Read the model definition and answer for the solid it produces. Units are mm, in the model's axes. A direction names the side the tool comes from. Give positions to 0.01 mm unless a question says otherwise; leave off trailing zeros. Loops run counter-clockwise (first coordinate to the right, second up) from the corner with the lowest first, then second, coordinate; pieces in that order, holes last. Notation, with made-up numbers: (9.5, 84) - (20.5, 84) arc R4 ccw to (20.5, 89) - close; hole circle Ø8 at (1.25, -39). An arc over 180 degrees is marked (long way). Use a Markdown table: item, result. Add a question column.
Item 1: A cutting plane is placed at D-D (y = -9.75). Determine the outline of the cut face in (x, z) (3 decimals).
Item 2: Each of these flat-tipped pins is pushed along its axis until it touches: P1, Ø1.5, axis at y = -3.5, z = -13, coming from the -X side; P2, Ø2, axis at x = 29.5, y = -4.5, coming from the -Z side; P3, Ø1.9, axis at x = 21, y = 4.5, coming from the -Z side. Where does it stop, or does it pass through?
Item 3: A cutting plane is placed at A-A (z = -11). Determine the outline of the cut face in (x, y), plus the area to 3 significant figures.
Item 4: A cutting plane is placed at B-B (z = -16.25). Determine the outline of the cut face in (x, y), plus the area to 3 significant figures.
Item 5: Consider probe 1 along X at (y, z) = (0.7, -3.5); probe 2 along X at (y, z) = (0.75, -0.75); probe 3 along Y at (x, z) = (25, -2.25). Determine where each line is inside the solid, lowest interval first. Write a range as [from, to].
Item 6: For a pull along Z with two mould halves and no side action, classify faces 1 (the face through (3.6, 0.8, -21.5)), 2 (the face through (1.05, 0.79, -21)), 3 (the face through (11.968, -6.039, -19.117)) as +Z half, -Z half, draft (parallel to the pull), parting line (faces both ways), or undercut.
Item 7: A cutting plane is placed at C-C (x = 37.5). Determine the outline of the cut face in (y, z).
Item 8: Which of the six approach directions +Z, -Z, +X, -X, +Y, -Y give full straight-line access (tool end or side, diameter ignored) to faces 4 (the face through (39.619, -6.039, -17.448)), 5 (the face through (23, 5, -5.5)), 6 (the face through (28.5, 5, -3))?
from build123d import *

# Parameters (mm, degrees)
SKETCH1_R           = 3
BOSS_EXTRUDE1_DEPTH = 1.6
SKETCH2_W           = 10
SKETCH2_H           = 5.5
BOSS_EXTRUDE2_DEPTH = 6.25
SKETCH3_R           = 8.125
BOSS_EXTRUDE3_DEPTH = 12.25


with BuildPart() as part:
    # Sketch1 → Boss-Extrude1 (new body)
    with BuildSketch(Plane(origin=(0, 0, 0), x_dir=(1, 0, 0), z_dir=(0, 1, 0))):
        with BuildLine():
            Line((3.5, 0), (43.5, 0))
            ThreePointArc((43.5, 0), (45.974873734, 1.025126266), (47, 3.5))
            Line((47, 3.5), (47, 18.5))
            ThreePointArc((47, 18.5), (45.974873734, 20.974873734), (43.5, 22))
            Line((43.5, 22), (3.5, 22))
            ThreePointArc((3.5, 22), (1.025126266, 20.974873734), (0, 18.5))
            Line((0, 18.5), (0, 3.5))
            ThreePointArc((0, 3.5), (1.025126266, 1.025126266), (3.5, 0))
        make_face()
        with Locations(Location((3.5, 18.5, 0), (0, 0, 270))):
            Circle(SKETCH1_R, mode=Mode.SUBTRACT)
        with Locations(Location((3.5, 3.5, 0), (0, 0, 270))):
            Circle(SKETCH1_R, mode=Mode.SUBTRACT)
        with Locations(Location((43.5, 3.5, 0), (0, 0, 270))):
            Circle(SKETCH1_R, mode=Mode.SUBTRACT)
        with Locations(Location((43.5, 18.5, 0), (0, 0, 270))):
            Circle(SKETCH1_R, mode=Mode.SUBTRACT)
    extrude(amount=BOSS_EXTRUDE1_DEPTH)

    # Sketch2 → Boss-Extrude2 (add)
    with BuildSketch(Plane(origin=(0, 1.6, 0), x_dir=(1, 0, 0), z_dir=(0, 1, 0))):
        with Locations((23.5, 2.75)):
            Rectangle(SKETCH2_W, SKETCH2_H)
    extrude(amount=BOSS_EXTRUDE2_DEPTH)

    # Sketch3 → Boss-Extrude3 (add)
    with BuildSketch(Plane(origin=(0, 0, 0), x_dir=(-1, 0, 0), z_dir=(0, -1, 0))):
        with Locations(Location((-12.325, 11, 0), (0, 0, 270))):
            Circle(SKETCH3_R)
        with Locations(Location((-34.675, 11, 0), (0, 0, 270))):
            Circle(SKETCH3_R)
    extrude(amount=BOSS_EXTRUDE3_DEPTH)


solid = part.part
Geometry says:
| question | item | result |
|---|---|---|
| 1 | outline | circle Ø16.25 at (12.325, -11); circle Ø16.25 at (34.675, -11) |
| 2 | P1 | x = 4.3 |
| 2 | P2 | z = -17.97 |
| 2 | P3 | z = -5.5 |
| 3 | outline | (0, 0) - (4.2, 0) - (4.2, -12.25) - (20.45, -12.25) - (20.45, 0) - (26.55, 0) - (26.55, -12.25) - (42.8, -12.25) - (42.8, 0) - (47, 0) - (47, 1.6) - (0, 1.6) - close |
| 3 | area | 473 mm² |
| 4 | outline | (0, 0) - (1.52, 0) - (1.52, 1.6) - (0, 1.6) - close; (5.48, 0) - (6.12, 0) - (6.12, -12.25) - (18.53, -12.25) - (18.53, 0) - (28.47, 0) - (28.47, -12.25) - (40.88, -12.25) - (40.88, 0) - (41.52, 0) - (41.52, 1.6) - (5.48, 1.6) - close; (45.48, 0) - (47, 0) - (47, 1.6) - (45.48, 1.6) - close |
| 4 | area | 366 mm² |
| 5 | probe 1 | [0, 0.5], [6.5, 40.5], [46.5, 47] |
| 5 | probe 2 | [1.33, 2.3], [4.7, 42.3], [44.7, 45.67] |
| 5 | probe 3 | [0, 7.85] |
| 6 | face 1 | undercut |
| 6 | face 2 | -Z half |
| 6 | face 3 | parting line |
| 7 | outline | (-12.25, -18.62) - (0, -18.62) - (0, -22) - (1.6, -22) - (1.6, 0) - (0, 0) - (0, -3.38) - (-12.25, -3.38) - close |
| 8 | face 4 | -Y |
| 8 | face 5 | -Z, +X, -X, +Y |
| 8 | face 6 | +Z, -Z, +X, +Y |
